Can you work these out from the model? Positions are in its coordinate system, mm. Face numbers are marked on the shaded views. A direction names the side the tool comes from. Give positions to 0.01 mm unless a question says otherwise; leave off trailing zeros. Order: outer loops, then holes, each group sorted by start corner. A loop starts at its lowest first (then second) coordinate and runs counter-clockwise, first axis right, second up. Notation, with made-up numbers: M -20,-11.5 L 17,-11.5 A21 ccw 17,25.5 Z; hole C 46,-9 d11. An arc over 180 degrees is marked long. Write each question's results on one line, items separated by ' | '.
from build123d import *

# Parameters (mm, degrees)
SKETCH_1_W          = 16
SKETCH_1_H          = 16
SKETCH_1_W_2        = 14
SKETCH_1_H_2        = 14
EXTRUDE_1_DEPTH     = 52
SKETCH_2_W          = 16
SKETCH_2_H          = 16
EXTRUDE_2_DEPTH     = 1
SKETCH_3_W          = 16
SKETCH_3_H          = 16
EXTRUDE_3_DEPTH     = 16
CUT_EXTRUDE_1_DEPTH = 16
SKETCH_5_W          = 16
SKETCH_5_H          = 8
CUT_EXTRUDE_2_DEPTH = 17


with BuildPart() as part:
    # 草图1 → 凸台-拉伸1 (new body)
    with BuildSketch(Plane.XY):
        Rectangle(SKETCH_1_W, SKETCH_1_H)
        Rectangle(SKETCH_1_W_2, SKETCH_1_H_2, mode=Mode.SUBTRACT)
    extrude(amount=EXTRUDE_1_DEPTH)

    # 草图2 → 凸台-拉伸2 (add)
    with BuildSketch(Plane(origin=(0, 0, 0), x_dir=(-1, 0, 0), z_dir=(0, 0, -1))):
        Rectangle(SKETCH_2_W, SKETCH_2_H)
    extrude(amount=EXTRUDE_2_DEPTH)

    # 草图3 → 凸台-拉伸3 (add)
    with BuildSketch(Plane(origin=(0, 0, -1), x_dir=(-1, 0, 0), z_dir=(0, 0, -1))):
        Rectangle(SKETCH_3_W, SKETCH_3_H)
    extrude(amount=EXTRUDE_3_DEPTH)

    # 草图4 → 切除-拉伸1 (cut)
    with BuildSketch(Plane.XZ.offset(8)):
        with BuildLine():
            Line((-8, -9), (-8, -21.563953952))
            Line((-8, -21.563953952), (8, -21.563953952))
            Line((8, -21.563953952), (8, -9))
            ThreePointArc((8, -9), (0, -17), (-8, -9))
        make_face()
    extrude(amount=-CUT_EXTRUDE_1_DEPTH, mode=Mode.SUBTRACT)

    # 草图5 → 切除-拉伸2 (cut, through all)
    with BuildSketch(Plane(origin=(8, 0, 0), x_dir=(0, 0, -1), z_dir=(1, 0, 0))):
        with Locations((9, 0)):
            Rectangle(SKETCH_5_W, SKETCH_5_H)
    extrude(amount=-CUT_EXTRUDE_2_DEPTH, mode=Mode.SUBTRACT)


solid = part.part
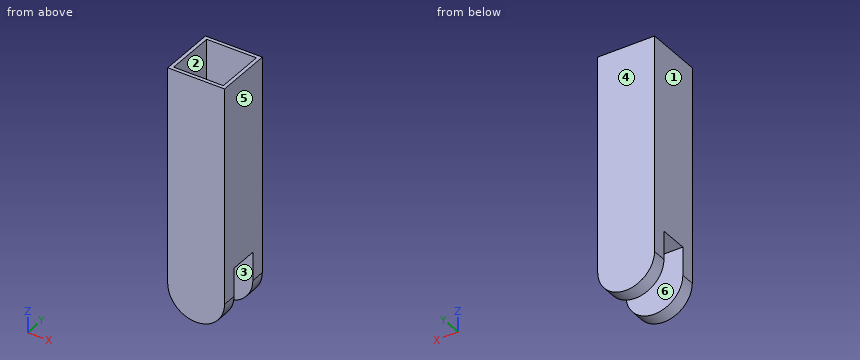
(1) We'd pull the mould along Y, two halves only. Please class the marked faces 4, 5 and 6: +Y half, -Y half, draft (parallel to the pull), parting line (faces both ways), or undercut.
Data:
face 4: +Y half | face 5: draft | face 6: undercut
(2) Imagine slicing it at C-C, the plane y = -2.25. Write out the boundary of the cut face in (x, z).
Data:
outline: M -8,-1 L 8,-1 L 8,52 L 7,52 L 7,0 L -7,0 L -7,52 L -8,52 Z
(3) I need wall thicknesses on L1, parallel to Y at x = 5.75, z = 33.5; L2, parallel to Y at x = 3.5, z = -6.5. Which ranges of each line are inside material? Lowest first, please. Write a range as from..to.
Data:
L1: y = -8..-7, 7..8 | L2: y = -8..-4, 4..8
(4) Imagine slicing it at D-D, the plane z = 18. Write out the boundary of the cut face in (x, y), plus the area to 3 significant figures.
Data:
outline: M -8,-8 L 8,-8 L 8,8 L -8,8 Z; hole M -7,-7 L 7,-7 L 7,7 L -7,7 Z | area: 60.0 mm2
(5) Imagine slicing it at A-A, the plane z = -5.5. Write out the boundary of the cut face in (x, y), plus the area to 3 significant figures.
Data:
outline: M -8,-8 L 8,-8 L 8,-4 L -8,-4 Z; M -8,4 L 8,4 L 8,8 L -8,8 Z | area: 128 mm2
(6) For the marked faces 1, 2 and 3, which set-ups out of +Z, -Z, +X, -X, +Y, -Y let a thin tool reach every point of the face, with its end or its side?
Data:
face 1: +Z, -Z, -X, +Y, -Y | face 2: +Z | face 3: -Z, +X, -X
(7) Will these pins go through, and if not, where does the flat tip stop? P1, Ø4, axis at x = -0.5, y = 0.5, coming from the -Z side; P2, Ø4, axis at x = 2, y = 1, coming from the +Z side.
Data:
P1: stops at z = -1 | P2: stops at z = 0
(8) Imagine slicing it at B-B, the plane x = 0. Write out the boundary of the cut face in (y, z).
Data:
outline: M -8,-17 L -4,-17 L -4,-1 L 4,-1 L 4,-17 L 8,-17 L 8,52 L 7,52 L 7,0 L -7,0 L -7,52 L -8,52 Z
